```python
from build123d import *

# Parameters (mm, degrees)
BOSS_EXTRUDE2_DEPTH  = 38
BOSS_EXTRUDE3_DEPTH  = 9
SKETCH5_R            = 9
BOSS_EXTRUDE4_DEPTH  = 40
CUT_EXTRUDE1_DEPTH   = 61
MIRROR2_COPY_1_DEPTH = 61
CUT_EXTRUDE3_DEPTH   = 40
SKETCH7_R            = 4.5
CUT_EXTRUDE4_DEPTH   = 61


with BuildPart() as part:
    # Sketch1 → Boss-Extrude2 (new body)
    with BuildSketch(Plane.XY):
        with BuildLine():
            Line((27, 0), (36, 0))
            ThreePointArc((36, 0), (0, -36), (-36, 0))
            Line((-36, 0), (-27, 0))
            Line((-27, 0), (27, 0))
        make_face()
    extrude(amount=BOSS_EXTRUDE2_DEPTH)

    # Sketch4 → Boss-Extrude3 (add, symmetric)
    with BuildSketch(Plane.XY.offset(19)):
        with BuildLine():
            Line((-36, 0), (-47, 0))
            Line((-47, 0), (-47, -40))
            Line((-47, -40), (-22, -60))
            Line((-22, -60), (22, -60))
            Line((22, -60), (47, -40))
            Line((47, -40), (47, 0))
            Line((47, 0), (36, 0))
            ThreePointArc((36, 0), (0, -36), (-36, 0))
        make_face()
    extrude(amount=BOSS_EXTRUDE3_DEPTH, both=True)

    # Sketch5 → Boss-Extrude4 (add)
    with BuildSketch(Plane(origin=(0, 0, 0), x_dir=(1, 0, 0), z_dir=(0, 1, 0))):
        with Locations((-38, -19)):
            Circle(SKETCH5_R)
        with Locations((38, -19)):
            Circle(SKETCH5_R)
    extrude(amount=-BOSS_EXTRUDE4_DEPTH)

    # Sketch6 → Cut-Extrude1 (cut, through all)
    with BuildSketch(Plane(origin=(0, 0, 0), x_dir=(1, 0, 0), z_dir=(0, 1, 0))):
        with BuildLine():
            Line((-47, -19), (-47, -10))
            Line((-47, -10), (-38, -10))
            ThreePointArc((-38, -10), (-44.363961031, -12.636038969), (-47, -19))
        make_face()
    cut_extrude1 = extrude(amount=-CUT_EXTRUDE1_DEPTH, mode=Mode.SUBTRACT)

    # Mirror1: Cut-Extrude1 across plane
    add(cut_extrude1.mirror(Plane.XY.offset(19)), mode=Mode.SUBTRACT)

    # Mirror2: Cut-Extrude1 across plane
    add(cut_extrude1.mirror(Plane(origin=(0, 0, 0), x_dir=(0, 0, 1), z_dir=(1, 0, 0))), mode=Mode.SUBTRACT)

    # Mirror2 copy 1 sketch → Mirror2 copy 1 (cut, through all)
    with BuildSketch(Plane(origin=(0, 0, 38), x_dir=(-1, 0, 0), z_dir=(0, 1, 0))):
        with BuildLine():
            Line((-47, -19), (-47, -10))
            Line((-47, -10), (-38, -10))
            ThreePointArc((-38, -10), (-44.363961031, -12.636038969), (-47, -19))
        make_face()
    extrude(amount=-MIRROR2_COPY_1_DEPTH, mode=Mode.SUBTRACT)

    # Sketch3 → Cut-Extrude3 (cut)
    with BuildSketch(Plane.XY.offset(38)):
        with BuildLine():
            Line((-27, 0), (27, 0))
            ThreePointArc((27, 0), (0, -27), (-27, 0))
        make_face()
    extrude(amount=-CUT_EXTRUDE3_DEPTH, mode=Mode.SUBTRACT)

    # Sketch7 → Cut-Extrude4 (cut, through all)
    with BuildSketch(Plane(origin=(0, 0, 0), x_dir=(1, 0, 0), z_dir=(0, 1, 0))):
        with Locations((-38, -19)):
            Circle(SKETCH7_R)
        with Locations((38, -19)):
            Circle(SKETCH7_R)
    extrude(amount=-CUT_EXTRUDE4_DEPTH, mode=Mode.SUBTRACT)


solid = part.part
```
CAD build for the part. Positions are in the model's coordinates, mm. A direction names the side the tool comes from. Round coordinates to 2 decimals unless told otherwise and drop trailing zeros. Loops run counter-clockwise (first coordinate to the right, second up) from the corner with the lowest first, then second, coordinate; pieces in that order, holes last. Notation, with made-up numbers: (-32, -19) - (18, -19) arc R29 ccw to (18, 11) - close; hole circle Ø5 at (38, 55.5). An arc over 180 degrees is marked (long way). Return JSON: item names as keys, results as strings. Group by question number.
Q1. Drill centre lines: line 1 along X through (y, z) = (-29, 19); line 2 along X through (y, z) = (-17.5, 22); line 3 along X through (y, z) = (-31, 17). Where is each one in solid material? Low to high. Write a range as [from, to].
Q2. Band-saw the part on C-C on y = -14.5. Give the cut face in (x, z).
Q3. Band-saw the part on A-A on y = -23.5. Give the cut face in (x, z), plus the area to 3 significant figures.
Q4. Band-saw the part on B-B on x = 0. Give the cut face in (y, z), plus the area to 3 significant figures.
Q5. Flat gauge pins, fed straight in: pin 1 Ø8 at (y, z) = (-38, 16) entering from -X; pin 2 Ø5 at (y, z) = (-38.5, 22.5) entering from +X; pin 3 Ø8 at (x, z) = (21, 33.5) entering from -Y; pin 4 Ø5.5 at (x, z) = (38, 19) entering from +Y. Where does each tip first touch, or does it go through?
Q6. Two-plate mould, pull along Z, no slides. Class faces 4 (the face through (0.2, -27.2, 0)), 5 (the face through (33.504, -25.118, 18.802)), 6 (the face through (32, 0, 19)): +Z half, -Z half, draft (parallel to the pull), parting line (faces both ways), or undercut.
Q7. Band-saw the part on D-D on z = 20.5. Give the cut face in (x, y), plus the area to 3 significant figures.
Q8. Tool access for faces 1 (the face through (-33, 0, 19)), 2 (the face through (0.79, -35.99, 32.93)), 3 (the face through (0.79, -35.99, 4.93)): list every direction of +Z, -Z, +X, -X, +Y, -Y with a clear straight run to the whole face (end or side of a thin tool).
Solutions:
{
 "1": {"line 1": "x = [-47, -42.5], [-33.5, 33.5], [42.5, 47]", "line 2": "x = [-46.49, -41.35], [-34.65, -20.56], [20.56, 34.65], [41.35, 46.49]", "line 3": "x = [-46.77, -42.03], [-33.97, 33.97], [42.03, 46.77]"},
 "2": {"outline": "(-38, 10) - (-32.95, 10) - (-32.95, 0) - (-22.78, 0) - (-22.78, 38) - (-32.95, 38) - (-32.95, 28) - (-38, 28) arc R9 ccw to start; (22.78, 0) - (32.95, 0) - (32.95, 10) - (38, 10) arc R9 ccw to (38, 28) - (32.95, 28) - (32.95, 38) - (22.78, 38) - close; hole circle Ø9 at (-38, 19); hole circle Ø9 at (38, 19)"},
 "3": {"outline": "(-38, 10) - (-27.27, 10) - (-27.27, 0) - (-13.29, 0) - (-13.29, 38) - (-27.27, 38) - (-27.27, 28) - (-38, 28) arc R9 ccw to start; (13.29, 0) - (27.27, 0) - (27.27, 10) - (38, 10) arc R9 ccw to (38, 28) - (27.27, 28) - (27.27, 38) - (13.29, 38) - close; hole circle Ø9 at (-38, 19); hole circle Ø9 at (38, 19)", "area": "1,580 mm^2"},
 "4": {"outline": "(-60, 10) - (-36, 10) - (-36, 0) - (-27, 0) - (-27, 38) - (-36, 38) - (-36, 28) - (-60, 28) - close", "area": "774 mm^2"},
 "5": {"pin 1": "stops at x = -47", "pin 2": "stops at x = 46.94", "pin 3": "stops at y = -31.73", "pin 4": "passes through"},
 "6": {"face 4": "-Z half", "face 5": "undercut", "face 6": "draft"},
 "7": {"outline": "(-46.87, -40.1) - (-42.24, -43.81) - (-42.24, 0) - (-46.87, 0) - close; (-33.76, -50.59) - (-22, -60) - (22, -60) - (33.76, -50.59) - (33.76, 0) - (27, 0) arc R27 cw to (-27, 0) - (-33.76, 0) - close; (42.24, -43.81) - (46.87, -40.1) - (46.87, 0) - (42.24, 0) - close", "area": "3,180 mm^2"},
 "8": {"face 1": "+Z, -Z, +X, -X, +Y", "face 2": "+Z, -Y", "face 3": "-Z, -Y"}
}
